The model under review builds one solid part; all positions refer to its coordinate system, in mm. Give positions to 0.01 mm unless a question says otherwise; leave off trailing zeros. Loops run counter-clockwise (first coordinate to the right, second up) from the corner with the lowest first, then second, coordinate; pieces in that order, holes last. Notation, with made-up numbers: M 57,-34.5 L 73,-34.5 A26 ccw 73,-15.5 Z; hole C 57,88 d9. An arc over 180 degrees is marked long. Return JSON: item names as keys, results as strings. Group by question number.
```python
from build123d import *

# Parameters (mm, degrees)
SKETCH1_W                    = 5.55625
SKETCH1_H                    = 9.525
BOSS_EXTRUDE1_DEPTH          = 107.95
SKETCH17_W                   = 1.651
SKETCH17_H                   = 2.667
CUT_EXTRUDE8_DEPTH           = 216.9
SKETCH18_W                   = 1.651
SKETCH18_H                   = 1.524
CUT_EXTRUDE9_DEPTH           = 216.9
F_18_0_1695_DIAMETER_HOLE1_D = 4.3053
CHAMFER1_SIZE                = 1.524
CHAMFER1_SIZE2               = 25.4
CHAMFER2_SIZE                = 25.4
CHAMFER2_SIZE2               = 1.524
SKETCH25_W                   = 1.7145
SKETCH25_H                   = 215.9
SKETCH25_W_2                 = 2.19075
BOSS_EXTRUDE2_DEPTH          = 3.175
CHAMFER3_SIZE                = 6.35


with BuildPart() as part:
    # Sketch1 → Boss-Extrude1 (new body, symmetric)
    with BuildSketch(Plane.XY):
        with Locations((2.778125, 0)):
            Rectangle(SKETCH1_W, SKETCH1_H)
    extrude(amount=BOSS_EXTRUDE1_DEPTH, both=True)

    # Sketch17 → Cut-Extrude8 (cut, through all)
    with BuildSketch(Plane.XY.offset(107.95)):
        with Locations((2.54, 3.429)):
            Rectangle(SKETCH17_W, SKETCH17_H)
    extrude(amount=-CUT_EXTRUDE8_DEPTH, mode=Mode.SUBTRACT)

    # Sketch18 → Cut-Extrude9 (cut, through all)
    with BuildSketch(Plane.XY.offset(107.95)):
        with Locations((3.0607, -4.0005)):
            Rectangle(SKETCH18_W, SKETCH18_H)
    extrude(amount=-CUT_EXTRUDE9_DEPTH, mode=Mode.SUBTRACT)

    # #18 (0.1695) Diameter Hole1 (through all)
    with Locations(Plane.ZY):
        with Locations((69.85, -0.396875), (-69.85, -0.396875), (0, -0.396875)):
            Hole(F_18_0_1695_DIAMETER_HOLE1_D / 2)

    # Chamfer1
    chamfer1_edges = [part.edges().sort_by_distance(p)[0] for p in [
        (2.54, 2.0955, 107.95),
    ]]
    chamfer1_side = [part.faces().sort_by_distance(p)[0] for p in [
        (2.785461813, -0.109400999, 107.95),
    ]]
    chamfer(chamfer1_edges, length=CHAMFER1_SIZE, length2=CHAMFER1_SIZE2, reference=chamfer1_side[0])

    # Chamfer2
    chamfer2_edges = [part.edges().sort_by_distance(p)[0] for p in [
        (2.54, 2.0955, -107.95),
    ]]
    chamfer2_side = [part.faces().sort_by_distance(p)[0] for p in [
        (2.54, 2.0955, -12.7),
    ]]
    chamfer(chamfer2_edges, length=CHAMFER2_SIZE, length2=CHAMFER2_SIZE2, reference=chamfer2_side[0])

    # Sketch25 → Boss-Extrude2 (add)
    with BuildSketch(Plane(origin=(0, 4.7625, 0), x_dir=(1, 0, 0), z_dir=(0, 1, 0))):
        with Locations((0.85725, 0)):
            Rectangle(SKETCH25_W, SKETCH25_H)
        with Locations((4.460875, 0)):
            Rectangle(SKETCH25_W_2, SKETCH25_H)
    extrude(amount=BOSS_EXTRUDE2_DEPTH)

    # Chamfer3
    chamfer3_edges = [part.edges().sort_by_distance(p)[0] for p in [
        (4.460875, 7.9375, -107.95),
        (4.460875, 7.9375, 107.95),
        (0.85725, 7.9375, 107.95),
        (0.85725, 7.9375, -107.95),
    ]]
    chamfer(chamfer3_edges, length=CHAMFER3_SIZE)


solid = part.part
```
(1) Mouldability with a two-part tool opening along Y and no side actions: class faces 1 (the cylindrical face through (2.817, 0.25, -71.903)), 2 (the flat face through (5.556, 1, 2)), 3 (the flat face through (0.85, 4.81, 104.73)) as released by +Y, released by -Y, zero draft, split by the parting line, or undercut.
(2) Add section B-B (z = 10). Write out the cut boundary in (x, y).
(3) For pin 1 (1.3 mm diameter, centred on x = 3, z = -29.5, fed in from -Y), flat-tipped, find the tip position at first contact; note if it passes through.
(4) Add section C-C (y = 6). Write out the cut boundary in (x, z).
(5) For probe 1 along Z at (x, y) = (3.65, -0.75); probe 2 along Y at (x, z) = (2.3, 69.85); probe 3 along X at (y, z) = (6.5, 94), list the stretches that pass through material, from the lowest coordinate up.
(6) Add section A-A (z = -69.85). Write out the cut boundary in (x, y).
Verdict:
{
 "1": {"face 1": "undercut", "face 2": "zero draft", "face 3": "released by +Y"},
 "2": {"outline": "M 0,-4.76 L 2.24,-4.76 L 2.24,-3.24 L 3.89,-3.24 L 3.89,-4.76 L 5.56,-4.76 L 5.56,7.94 L 3.37,7.94 L 3.37,2.1 L 1.71,2.1 L 1.71,7.94 L 0,7.94 Z"},
 "3": {"pin 1": "stops at y = -3.24"},
 "4": {"outline": "M 0,-103.54 L 1.71,-103.54 L 1.71,103.54 L 0,103.54 Z; M 3.37,-103.54 L 5.56,-103.54 L 5.56,103.54 L 3.37,103.54 Z"},
 "5": {"probe 1": "z = -107.95 to -71.97, -67.73 to -2.12, 2.12 to 67.73, 71.97 to 107.95", "probe 2": "y = -3.24 to -2.55, 1.76 to 2.1", "probe 3": "x = 0 to 1.71, 3.37 to 5.56"},
 "6": {"outline": "M 0,-4.76 L 2.24,-4.76 L 2.24,-3.24 L 3.89,-3.24 L 3.89,-4.76 L 5.56,-4.76 L 5.56,-2.55 L 0,-2.55 Z; M 0,1.76 L 5.56,1.76 L 5.56,7.94 L 3.37,7.94 L 3.37,2.1 L 1.71,2.1 L 1.71,7.94 L 0,7.94 Z"}
}
